Geometry check sheet. Reference: the model listing, model coordinates, mm. Face numbers are marked on the shaded views. A direction names the side the tool comes from. Give positions to 0.01 mm unless a question says otherwise; leave off trailing zeros. Order: outer loops, then holes, each group sorted by start corner. A loop starts at its lowest first (then second) coordinate and runs counter-clockwise, first axis right, second up. Notation, with made-up numbers: M 50.25,22 L 85.25,22 A22 cw 85.25,44 Z; hole C 15,57 d1. An arc over 180 degrees is marked long. Put each result on its own line as item: value. Start each with the question number.
Q1. Material ranges on L1, parallel to Z at x = 62.4, y = -40.6; L2, parallel to X at y = -43.5, z = -18.5; L3, parallel to Y at x = 62.45, z = 15.6, recorded low to high.
Q2. Mould release check, pull along Z, two halves, no side actions. Record for the marked faces 1, 2 and 3: +Z half, -Z half, draft (parallel to the pull), parting line (faces both ways), or undercut.
Q3. Section check A-A on y = -12.5. Record the cut outline in (x, z).
Q4. Section check B-B on x = 35. Record the cut outline in (y, z).
Q5. Go/stop test with flat-tipped pins: pin 1 (2.5 mm diameter, centred on y = -40.6, z = 15.6, fed in from +X); pin 2 (1.6 mm diameter, centred on x = 45.5, z = -4.5, fed in from +Y); pin 3 (2 mm diameter, centred on x = -38.5, z = -0.5, fed in from -Y). Record where each tip stops, or that it passes through.
Q6. Access from +Z, -Z, +X, -X, +Y, -Y to the whole of each face (thin tool, end or side, straight path). Record for the marked faces 4 and 5.
Q7. Section check C-C on z = -12.5. Record the cut outline in (x, y), then the cut area to 3 significant figures.
```python
from build123d import *

# Parameters (mm, degrees)
F0_W           = 127
F0_H           = 50
F1_DEPTH       = 50
F3_DEPTH       = 42
F4_R           = 11
F5_DEPTH       = 5
F7_DEPTH       = 15
F8_T2_ANGLE    = 343.7894292622
F9_R           = 5
F12_W          = 40
F12_H          = 42
F13_DEPTH      = 46
F14_R          = 1.6
F15_DEPTH      = 1
F16_R          = 1
F17_DEPTH      = 2
F17_DEPTH_BACK = 1.03
F18_DEPTH      = 25
F19_DEPTH      = 2
F20_DEPTH      = 25
F22_DEPTH      = 8
F23_R          = 2.8130076525
F24_DEPTH      = 3
F25_R          = 0.5
F26_R          = 11
F27_DEPTH      = 5


# Not quite as in the source:
# - a fillet or chamfer that OpenCascade refuses, or shapes differently, is made with other operations: its cross-section is extruded or revolved along the edge and cut away or added


with BuildPart() as f1:
    # F0 (on Front) → F1 (new body)
    with BuildSketch(Plane.XZ):
        Rectangle(F0_W, F0_H)
    extrude(amount=F1_DEPTH)

    # F2 (on face) → F3 (cut)
    with BuildSketch(Plane.YZ.offset(63.5)):
        Polygon((-41.7573593129, 21), (-46, 16.7573593129), (-46, -16.7573593129), (-41.7573593129, -21), (-8.2426406871, -21), (-4, -16.7573593129), (-4, 16.7573593129), (-8.2426406871, 21), align=None)
    extrude(amount=-F3_DEPTH, mode=Mode.SUBTRACT)

    # F4 (on face) → F5 (cut)
    with BuildSketch(Plane.XZ.offset(50)):
        with Locations((-38.5, 0)):
            Circle(F4_R)
    extrude(amount=-F5_DEPTH, mode=Mode.SUBTRACT)

    # F6 (on face) → F7 (cut)
    with BuildSketch(Plane.XZ.offset(45)):
        with BuildLine():
            Line((-37, 2), (-40, 2))
            ThreePointArc((-40, 2), (-38.5, -2.5), (-37, 2))
        make_face()
    extrude(amount=-F7_DEPTH, mode=Mode.SUBTRACT)

    # F8: fillet of radius 0.5 on 1 edges, made by hand

    # F8_s1 → F8_t2 (revolve)
    with BuildSketch(Plane(origin=(-37.7346622942, 0, -5.3739891953), x_dir=(0, 1, 0), z_dir=(0.9900106558, 0, 0.1409925581))):
        with BuildLine():
            ThreePointArc((-30.5, 7.9282134883), (-30.1464466094, 7.7817668789), (-30, 7.4282134883))
            Line((-30, 7.4282134883), (-30, 7.9282134883))
            Line((-30, 7.9282134883), (-30.5, 7.9282134883))
        make_face()
    revolve(axis=Axis((-38.5, -30, 0), (0, -1, 0)), revolution_arc=F8_T2_ANGLE)

    # F9
    f9_edges = [f1.edges().sort_by_distance(p)[0] for p in [
        (0, -50, 25),
        (0, -50, -25),
        (0, 0, 25),
        (0, 0, -25),
        (-63.5, -25, 25),
        (-63.5, -25, -25),
        (-63.5, 0, 0),
        (-63.5, -50, 0),
    ]]
    fillet(f9_edges, radius=F9_R)

    # F12 (on face) → F13 (cut)
    with BuildSketch(Plane.XZ.offset(50)):
        with Locations((41.5, 0)):
            Rectangle(F12_W, F12_H)
    extrude(amount=-F13_DEPTH, mode=Mode.SUBTRACT)

    # F14 (on face) → F15 (cut)
    with BuildSketch(Plane(origin=(0, 0, 0), x_dir=(-1, 0, 0), z_dir=(0, 1, 0))):
        with Locations((-46.0031795697, -4.1205275279)):
            Circle(F14_R)
        with Locations((-22.6282365388, 5.5031795697)):
            Circle(F14_R)
    extrude(amount=-F15_DEPTH, mode=Mode.SUBTRACT)

    # F16 (on face) → F17 (cut, two sides)
    with BuildSketch(Plane(origin=(0, 0, 2), x_dir=(1, 0, 0), z_dir=(0, 0, -1))) as f17_sk:
        Polygon((-36.5, 38.9047005384), (-38.5, 40.0594010768), (-40.5, 38.9047005384), (-40.5, 36.5952994616), (-38.5, 35.4405989232), (-36.5, 36.5952994616), align=None)
        with Locations((-38.5, 37.75)):
            Circle(F16_R, mode=Mode.SUBTRACT)
    extrude(amount=-F17_DEPTH, mode=Mode.SUBTRACT)
    extrude(f17_sk.sketch, amount=F17_DEPTH_BACK, mode=Mode.SUBTRACT)

    # F18 (cut): a face of the model
    f18_faces = [f1.faces().sort_by_distance(p)[0] for p in [
        (-38.5, -37.75, 2),
    ]]
    extrude(f18_faces, amount=-F18_DEPTH, mode=Mode.SUBTRACT)

    # F10 (on face) → F19 (join)
    with BuildSketch(Plane.YZ.offset(63.5)):
        Polygon((-46, 16.7573593129), (-46, -16.7573593129), (-41.7573593129, -21), (-8.2426406871, -21), (-4, -16.7573593129), (-4, 16.7573593129), (-8.2426406871, 21), (-16.9, 21), (-33.1, 21), (-41.7573593129, 21), align=None)
        with BuildLine():
            Line((-10.9, -15.6), (-39.1, -15.6))
            ThreePointArc((-39.1, -15.6), (-41.6606601718, -16.6606601718), (-40.6, -14.1))
            Line((-40.6, -14.1), (-40.6, 14.1))
            ThreePointArc((-40.6, 14.1), (-41.6606601718, 16.6606601718), (-39.1, 15.6))
            Line((-39.1, 15.6), (-10.9, 15.6))
            ThreePointArc((-10.9, 15.6), (-9.4, 17.1), (-7.9, 15.6))
            ThreePointArc((-7.9, 15.6), (-8.3393398282, 14.5393398282), (-9.4, 14.1))
            Line((-9.4, 14.1), (-9.4, -14.1))
            ThreePointArc((-9.4, -14.1), (-8.3393398282, -14.5393398282), (-7.9, -15.6))
            ThreePointArc((-7.9, -15.6), (-9.4, -17.1), (-10.9, -15.6))
        make_face(mode=Mode.SUBTRACT)
        with BuildLine():
            ThreePointArc((-40.6, -14.1), (-39.5393398282, -14.5393398282), (-39.1, -15.6))
            Line((-39.1, -15.6), (-10.9, -15.6))
            ThreePointArc((-10.9, -15.6), (-10.4606601718, -14.5393398282), (-9.4, -14.1))
            Line((-9.4, -14.1), (-9.4, 14.1))
            ThreePointArc((-9.4, 14.1), (-10.4606601718, 14.5393398282), (-10.9, 15.6))
            Line((-10.9, 15.6), (-39.1, 15.6))
            ThreePointArc((-39.1, 15.6), (-39.5393398282, 14.5393398282), (-40.6, 14.1))
            Line((-40.6, 14.1), (-40.6, -14.1))
        make_face()
    extrude(amount=-F19_DEPTH)

    # F11 (on face) → F20 (cut)
    with BuildSketch(Plane.YZ.offset(63.5)):
        with BuildLine():
            Line((-50, -11), (-25, -11))
            ThreePointArc((-25, -11), (-14, 0), (-25, 11))
            Line((-25, 11), (-50, 11))
            Line((-50, 11), (-50, -11))
        make_face()
    extrude(amount=-F20_DEPTH, mode=Mode.SUBTRACT)

    # F21 (on face) → F22 (cut)
    with BuildSketch(Plane.XZ.offset(45)):
        with BuildLine():
            Line((-35.85425, 3.0000011562), (-41.14575, 3.0000011562))
            ThreePointArc((-41.14575, 3.0000011562), (-38.5, -4), (-35.85425, 3.0000011562))
        make_face()
    extrude(amount=-F22_DEPTH, mode=Mode.SUBTRACT)

    # F23 (on face) → F24 (join)
    with BuildSketch(Plane.XZ.offset(37)):
        with Locations((-38.5, 0)):
            Circle(F23_R)
    extrude(amount=-F24_DEPTH)

    # F25
    f25_edges = [f1.edges().sort_by_distance(p)[0] for p in [
        (-38.5, -37, -4),
    ]]
    fillet(f25_edges, radius=F25_R)

    # F26 (on face) → F27 (join, through all)
    with BuildSketch(Plane.XZ.offset(45)):
        with Locations((-38.5, 0)):
            Circle(F26_R)
        with BuildLine():
            ThreePointArc((-35.85425, 3.0000011562), (-38.5, -4), (-41.14575, 3.0000011562))
            Line((-41.14575, 3.0000011562), (-35.85425, 3.0000011562))
        make_face(mode=Mode.SUBTRACT)
    extrude(amount=F27_DEPTH)


solid = f1.part
```
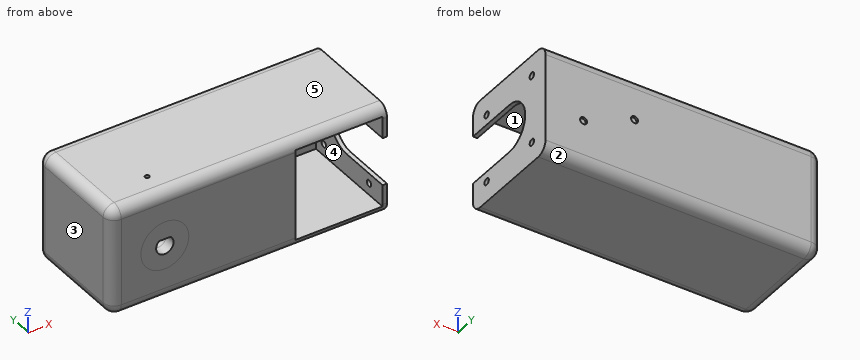
Results found:
1. L1: z = -25 to -17.1, -14.1 to -11, 11 to 14.1, 17.1 to 25
1. L2: x = -63.5 to 21.5, 61.5 to 63.5
1. L3: y = -50 to -42.1, -39.1 to -10.9, -7.9 to 0
2. face 1: undercut
2. face 2: -Z half
2. face 3: draft
3. outline: M -63.5,-20 A5 ccw -58.5,-25 L 63.5,-25 L 63.5,25 L -58.5,25 A5 ccw -63.5,20 Z; hole M 21.5,-21 L 61.5,-21 L 61.5,21 L 21.5,21 Z
4. outline: M -49.9,-21 A5 ccw -45,-25 L -5,-25 A5 ccw 0,-20 L 0,20 A5 ccw -5,25 L -45,25 A5 ccw -49.9,21 L -4,21 L -4,-21 Z
5. pin 1: stops at x = 21.5
5. pin 2: stops at y = -1
5. pin 3: stops at y = -37
6. face 4: -Y
6. face 5: +Z, +X, -X, +Y, -Y
7. outline: M -63.5,-45 A5 ccw -58.5,-50 L 21.5,-50 L 21.5,-4 L 61.5,-4 L 61.5,-50 L 63.5,-50 L 63.5,0 L -58.5,0 A5 ccw -63.5,-5 Z
7. area: 4,500 mm^2
